For this review, take the finished solid that the model builds, in its own axes (mm). Face numbers are marked on the shaded views. Coordinates: 2 decimals unless noted, no trailing zeros. Write each loop counter-clockwise with the first axis right and the second up, starting at its lowest first coordinate (ties: lowest second). Pieces come first, ordered by that corner, then holes. Notation, with made-up numbers: (9.5, 1.5) - (41.5, 1.5) arc R20 cw to (41.5, 36.5) - close; hole circle Ø2 at (70, 82). An arc over 180 degrees is marked (long way). Use one line per item in the form item = value. Start each with the question number.
1) We need section C-C (y = 7.25). Give the boundary of the cut face in (x, z).
2) For L1, parallel to Y at x = -16.5, z = -3; L2, parallel to X at y = 4, z = -10; L3, parallel to X at y = 2.5, z = 12, list the stretches that pass through material, from the lowest coordinate up. Write a range as from..to.
3) Insertion check: P1, Ø5, axis at x = -1, z = -7.5, coming from the +Y side; P2, Ø4, axis at x = 0, z = 8, coming from the -Y side; P3, Ø3, axis at x = 0, z = 8, coming from the +Y side. Each pin has a flat end and moves straight along its axis. Give the tip position at first contact, or say it passes through.
4) We need section A-A (z = 0). Count the separate pieces of the cut face and the enclosed holes in it, plus the area to 3 significant figures.
5) Mouldability with a two-part tool opening along X and no side actions: class the marked faces 1 and 2 as pulls with the +X half, pulls with the -X half, needs draft (parallel to the pull), parting line crosses it, or undercut.
```python
from build123d import *

# Parameters (mm, degrees)
SKETCH1_R                      = 21
BOSS_EXTRUDE1_DEPTH            = 5
FILLET1_R                      = 2.5
SKETCH2_R                      = 3
BOSS_EXTRUDE2_DEPTH            = 7.5
CBORE_FOR_M3_SHCS1_D           = 3.4
CBORE_FOR_M3_SHCS1_CBORE_D     = 6.5
CBORE_FOR_M3_SHCS1_CBORE_DEPTH = 3
CIRPATTERN1_COUNT              = 4


with BuildPart() as part:
    # Sketch1 → Boss-Extrude1 (new body)
    with BuildSketch(Plane(origin=(0, 0, 0), x_dir=(1, 0, 0), z_dir=(0, 1, 0))):
        with Locations(Location((0, 0, 0), (0, 0, 270))):
            Circle(SKETCH1_R)
    extrude(amount=BOSS_EXTRUDE1_DEPTH)

    # Fillet1
    fillet1_edges = [part.edges().sort_by_distance(p)[0] for p in [
        (0, 0, -21),
        (0, 5, -21),
    ]]
    fillet(fillet1_edges, radius=FILLET1_R - 0.0001)  # a hair under: the kernel refuses the full size

    # Sketch2 → Boss-Extrude2 (add)
    with BuildSketch(Plane(origin=(0, 5, 0), x_dir=(1, 0, 0), z_dir=(0, 1, 0))):
        with Locations(Location((-15.314964139, -2.387859588, 0), (0, 0, 188.862019992))):
            Circle(SKETCH2_R)
    extrude(amount=BOSS_EXTRUDE2_DEPTH)

    # CBORE for M3 SHCS1 (through all)
    with Locations(Plane(origin=(0, 5, 0), x_dir=(1, 0, 0), z_dir=(0, 1, 0))):
        with Locations((0, 0)):
            CounterBoreHole(CBORE_FOR_M3_SHCS1_D / 2, CBORE_FOR_M3_SHCS1_CBORE_D / 2, CBORE_FOR_M3_SHCS1_CBORE_DEPTH)

    # Sketch10 → CBORe for M2 (revolve, cut)
    with BuildSketch(Plane.XY, mode=Mode.PRIVATE) as cbore_for_m2_sk:
        Polygon((8, 5), (8, 0), (9.2, 0), (9.2, 3), (10.2, 3), (10.2, 5), align=None)
    cbore_for_m2 = revolve(cbore_for_m2_sk.sketch.rotate(Axis((8, 5, 0), (0, -1, 0)), 90), axis=Axis((8, 5, 0), (0, -1, 0)), mode=Mode.SUBTRACT)

    # CirPattern1: CBORe for M2 ×4 about axis
    cirpattern1_axis = Axis((0, 0, 0), (0, 1, 0))
    for i in range(1, CIRPATTERN1_COUNT):
        add(cbore_for_m2.rotate(cirpattern1_axis, i * 360 / CIRPATTERN1_COUNT), mode=Mode.SUBTRACT)


solid = part.part
```
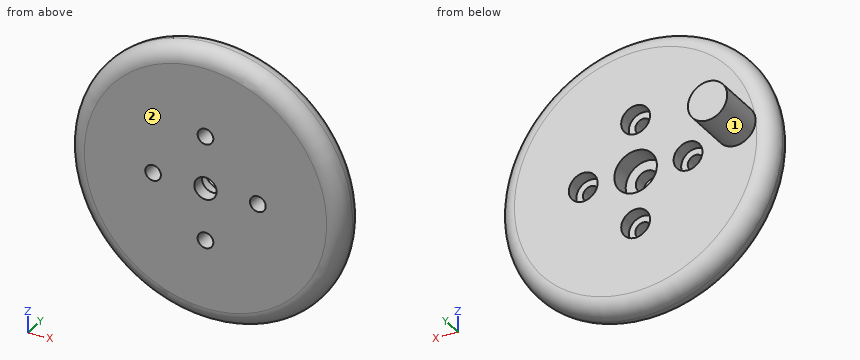
Determined:
q1.outline = circle Ø6 at (-15.31, 2.39)
q2.L1 = 0..5
q2.L2 = -17.9..-0.92, 0.92..17.9
q2.L3 = -17.23..17.23
q3.P1 = 5
q3.P2 = 0
q3.P3 = 3
q4.separate_pieces = 4
q4.enclosed_holes = 0
q4.area = 174 mm²
q5.face_1 = parting line crosses it
q5.face_2 = needs draft
